Work out the finished part from the listing and answer in its coordinate system (mm). Face numbers are marked on the shaded views. A direction names the side the tool comes from. Coordinates: 2 decimals unless noted, no trailing zeros. Write each loop counter-clockwise with the first axis right and the second up, starting at its lowest first coordinate (ties: lowest second). Pieces come first, ordered by that corner, then holes. Notation, with made-up numbers: (73, 20) - (131, 20) arc R15 ccw to (131, 39) - close; hole circle Ø6 at (20, 30). An arc over 180 degrees is marked (long way). Answer as a JSON object with one key per item and string values. Group by question number.
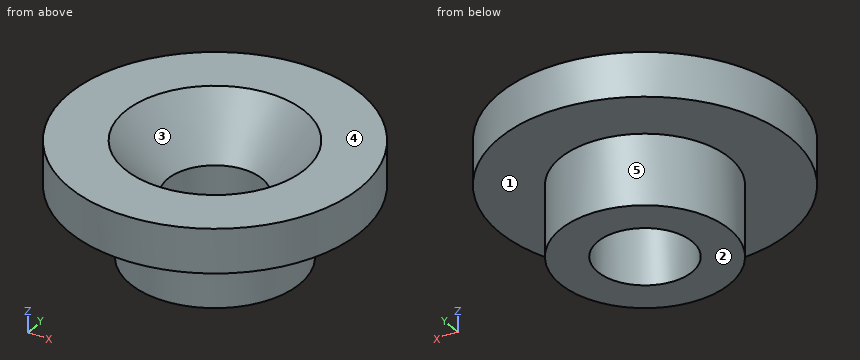
from build123d import *

# Parameters (mm, degrees)
SKETCH1_R           = 4.8
BOSS_EXTRUDE1_DEPTH = 4
SKETCH2_R           = 8.25
BOSS_EXTRUDE2_DEPTH = 2.5
SKETCH3_R           = 2.675
CUT_EXTRUDE1_DEPTH  = 6.5
SKETCH4_R           = 5.1
CUT_EXTRUDE2_DEPTH  = 3
CUT_EXTRUDE2_TAPER  = 39


with BuildPart() as part:
    # Sketch1 → Boss-Extrude1 (new body)
    with BuildSketch(Plane.XY):
        Circle(SKETCH1_R)
    extrude(amount=BOSS_EXTRUDE1_DEPTH)

    # Sketch2 → Boss-Extrude2 (add)
    with BuildSketch(Plane.XY.offset(4)):
        Circle(SKETCH2_R)
    extrude(amount=BOSS_EXTRUDE2_DEPTH)

    # Sketch3 → Cut-Extrude1 (cut)
    with BuildSketch(Plane.XY.offset(6.5)):
        Circle(SKETCH3_R)
    extrude(amount=-CUT_EXTRUDE1_DEPTH, mode=Mode.SUBTRACT)

    # Sketch4 → Cut-Extrude2 (cut)
    with BuildSketch(Plane.XY.offset(6.5)):
        Circle(SKETCH4_R)
    extrude(amount=-CUT_EXTRUDE2_DEPTH, taper=CUT_EXTRUDE2_TAPER, mode=Mode.SUBTRACT)


solid = part.part
Q1. A tool of negligible diameter and unlimited length cuts with its end or side. For the marked faces 1 and 2, from which of +Z, -Z, +X, -X, +Y, -Y can it reach the whole face along a straight path? Write none if from no direction.
Q2. Flat-ended cylindrical pins translate along their axes: pin 1 Ø3 at (y, z) = (-5, 5) entering from +X; pin 2 Ø2 at (x, y) = (-2, 6) entering from -Z; pin 3 Ø8.5 at (x, y) = (0, 0) entering from +Z. Find the tip coordinate at first contact, or state that the pin passes through.
Q3. Section A-A on x = 0 is taken. Determine the outline of the cut face in (y, z) (3 decimals).
Q4. For a pull along Y with two mould halves and no side action, classify the marked faces 3, 4 and 5 as +Y half, -Y half, draft (parallel to the pull), parting line (faces both ways), or undercut.
Q5. Consider L1, parallel to Y at x = 0, z = 2.35 (3 decimals); L2, parallel to X at y = -0.5, z = 4.75; L3, parallel to Y at x = 2, z = 0.5. Determine where each line is inside the solid, lowest interval first. Write a range as from..to.
Q6. Section B-B on z = 1.5 is taken. Determine the outline of the cut face in (x, y) (3 decimals).
Q7. Section D-D on z = 5.5 is taken. Determine the outline of the cut face in (x, y), plus the area to 3 significant figures.
Q8. Section C-C on y = -6.75 is taken. Determine the outline of the cut face in (x, z).
Numbers:
{
 "1": {"face 1": "-Z", "face 2": "-Z, +X, -X, +Y, -Y"},
 "2": {"pin 1": "stops at x = 7.47", "pin 2": "stops at z = 4", "pin 3": "stops at z = 5.45"},
 "3": {"outline": "(-8.25, 4) - (-4.8, 4) - (-4.8, 0) - (-2.675, 0) - (-2.675, 3.505) - (-5.1, 6.5) - (-8.25, 6.5) - close; (2.675, 0) - (4.8, 0) - (4.8, 4) - (8.25, 4) - (8.25, 6.5) - (5.1, 6.5) - (2.675, 3.505) - close"},
 "4": {"face 3": "undercut", "face 4": "draft", "face 5": "parting line"},
 "5": {"L1": "y = -4.8..-2.675, 2.675..4.8", "L2": "x = -8.23..-3.65, 3.65..8.23", "L3": "y = -4.36..-1.78, 1.78..4.36"},
 "6": {"outline": "circle Ø9.6 at (0, 0); hole circle Ø5.35 at (0, 0)"},
 "7": {"outline": "circle Ø16.5 at (0, 0); hole circle Ø8.58 at (0, 0)", "area": "156 mm²"},
 "8": {"outline": "(-4.74, 4) - (4.74, 4) - (4.74, 6.5) - (-4.74, 6.5) - close"}
}
